```python
from build123d import *
from OCP.BRepAlgoAPI import BRepAlgoAPI_Cut
from OCP.TopTools import TopTools_ListOfShape

# Parameters (mm, degrees)
BOSS_EXTRUDE1_DEPTH   = 8
CUT_EXTRUDE2_DEPTH    = 3.1
CUT_EXTRUDE4_DEPTH    = 3.1
CUT_EXTRUDE6_START    = -3.1
CUT_EXTRUDE6_DEPTH    = 3.1
CUT_EXTRUDE7_START    = -3.1
CUT_EXTRUDE7_DEPTH    = 3.1
FILLET1_R             = 0.1
BODY_MOVE_COPY1_ANGLE = 89
BODY_MOVE_COPY3_ANGLE = 1
CUT_EXTRUDE8_DEPTH    = 19.406951047
CUT_EXTRUDE9_DEPTH    = 19.406951047
SKETCH20_W            = 16
SKETCH20_H            = 7.8
BOSS_EXTRUDE2_DEPTH   = 2.54
BOSS_EXTRUDE3_DEPTH   = 16


with BuildPart() as part:
    # Sketch1 → Boss-Extrude1 (new body)
    with BuildSketch(Plane.XY.offset(4)):
        with BuildLine():
            Line((-3.6, 0), (-3.6, -16))
            ThreePointArc((-3.6, -16), (0, -19.6), (3.6, -16))
            Line((3.6, -16), (3.6, 0))
            ThreePointArc((3.6, 0), (0, 3.6), (-3.6, 0))
        make_face()
    extrude(amount=-BOSS_EXTRUDE1_DEPTH)

    # Sketch3 → Cut-Extrude2 (cut)
    with BuildSketch(Plane.XY.offset(4)):
        with BuildLine():
            Line((2.8, -4.8), (2.8, -3.2))
            ThreePointArc((2.8, -3.2), (2.578885438, -2.842229124), (2.16, -2.88))
            ThreePointArc((2.16, -2.88), (0, -3.6), (-2.16, -2.88))
            ThreePointArc((-2.16, -2.88), (-2.578885438, -2.842229124), (-2.8, -3.2))
            Line((-2.8, -3.2), (-2.8, -4.8))
            ThreePointArc((-2.8, -4.8), (-2.578885438, -5.157770876), (-2.16, -5.12))
            ThreePointArc((-2.16, -5.12), (0, -4.4), (2.16, -5.12))
            ThreePointArc((2.16, -5.12), (2.578885438, -5.157770876), (2.8, -4.8))
        make_face()
    extrude(amount=-CUT_EXTRUDE2_DEPTH, mode=Mode.SUBTRACT)

    # Sketch5 → Cut-Extrude4 (cut)
    with BuildSketch(Plane.XY.offset(4)):
        with BuildLine():
            Line((2.8, -12.8), (2.8, -11.2))
            ThreePointArc((2.8, -11.2), (2.578885438, -10.842229124), (2.16, -10.88))
            ThreePointArc((2.16, -10.88), (0, -11.6), (-2.16, -10.88))
            ThreePointArc((-2.16, -10.88), (-2.578885438, -10.842229124), (-2.8, -11.2))
            Line((-2.8, -11.2), (-2.8, -12.8))
            ThreePointArc((-2.8, -12.8), (-2.578885438, -13.157770876), (-2.16, -13.12))
            ThreePointArc((-2.16, -13.12), (0, -12.4), (2.16, -13.12))
            ThreePointArc((2.16, -13.12), (2.578885438, -13.157770876), (2.8, -12.8))
        make_face()
    extrude(amount=-CUT_EXTRUDE4_DEPTH, mode=Mode.SUBTRACT)

    # Sketch7 → Cut-Extrude6 (cut)
    with BuildSketch(Plane(origin=(0, 0, -4), x_dir=(-1, 0, 0), z_dir=(0, 0, -1)).offset(CUT_EXTRUDE6_START)):
        with BuildLine():
            Line((2.8, -4.8), (2.8, -3.2))
            ThreePointArc((2.8, -3.2), (2.578885438, -2.842229124), (2.16, -2.88))
            ThreePointArc((2.16, -2.88), (0, -3.6), (-2.16, -2.88))
            ThreePointArc((-2.16, -2.88), (-2.578885438, -2.842229124), (-2.8, -3.2))
            Line((-2.8, -3.2), (-2.8, -4.8))
            ThreePointArc((-2.8, -4.8), (-2.578885438, -5.157770876), (-2.16, -5.12))
            ThreePointArc((-2.16, -5.12), (0, -4.4), (2.16, -5.12))
            ThreePointArc((2.16, -5.12), (2.578885438, -5.157770876), (2.8, -4.8))
        make_face()
    extrude(amount=CUT_EXTRUDE6_DEPTH, mode=Mode.SUBTRACT)

    # Sketch8 → Cut-Extrude7 (cut)
    with BuildSketch(Plane(origin=(0, 0, -4), x_dir=(-1, 0, 0), z_dir=(0, 0, -1)).offset(CUT_EXTRUDE7_START)):
        with BuildLine():
            Line((-2.8, -11.2), (-2.8, -12.8))
            ThreePointArc((-2.8, -12.8), (-2.578885438, -13.157770876), (-2.16, -13.12))
            ThreePointArc((-2.16, -13.12), (0, -12.4), (2.16, -13.12))
            ThreePointArc((2.16, -13.12), (2.578885438, -13.157770876), (2.8, -12.8))
            Line((2.8, -12.8), (2.8, -11.2))
            ThreePointArc((2.8, -11.2), (2.578885438, -10.842229124), (2.16, -10.88))
            ThreePointArc((2.16, -10.88), (0, -11.6), (-2.16, -10.88))
            ThreePointArc((-2.16, -10.88), (-2.578885438, -10.842229124), (-2.8, -11.2))
        make_face()
    extrude(amount=CUT_EXTRUDE7_DEPTH, mode=Mode.SUBTRACT)

    # Sketch10 → Cut-Revolve1 (revolve, cut)
    with BuildSketch(Plane(origin=(0, -16, 0), x_dir=(1, 0, 0), z_dir=(0, 1, 0))):
        Polygon((3.1, 4), (0, 4), (0, -4), (3.1, -4), (3.1, -3.2), (2.4, -3.2), (2.4, 3.2), (3.1, 3.2), align=None)
    revolve(axis=Axis((0, -16, -4), (0, 0, 1)), mode=Mode.SUBTRACT)

    # Sketch13 → Cut-Revolve4 (revolve, cut)
    with BuildSketch(Plane(origin=(0, 0, 0), x_dir=(1, 0, 0), z_dir=(0, 1, 0))):
        Polygon((3.1, 4), (0, 4), (0, -4), (3.1, -4), (3.1, -3.2), (2.4, -3.2), (2.4, 3.2), (3.1, 3.2), align=None)
    revolve(axis=Axis((0, 0, -4), (0, 0, 1)), mode=Mode.SUBTRACT)

    # Fillet1
    fillet1_edges = [part.edges().sort_by_distance(p)[0] for p in [
        (0, -19.6, -4),
        (3.6, -8, -4),
        (0, 3.6, -4),
        (3.6, -8, 4),
        (0, -19.6, 4),
        (-3.6, -8, 4),
        (0, 3.6, 4),
        (-3.6, -8, -4),
    ]]
    fillet(fillet1_edges, radius=FILLET1_R)


with BuildPart() as part_1:
    # Body-Move/Copy1: moved
    add(part.part.rotate(Axis((-1.61875778, -8, 0), (0, 0, 1)), BODY_MOVE_COPY1_ANGLE))


with BuildPart() as part_2:
    # Body-Move/Copy3: read off the stored shape, not the designer's step
    # Body-Move/Copy3: moved
    add(part_1.part.moved(Location((-0.0519755, -0.1124913, 0))).rotate(Axis((0, 0, 0), (0, 0, 1)), BODY_MOVE_COPY3_ANGLE))

    # Sketch14 → Cut-Extrude8 (cut, through all)
    with BuildSketch(Plane.XY.offset(4)):
        Polygon((-3.814896337, -5.759656314), (-3.814896337, -7.283656314), (-2.290892666, -7.283656314), (-2.290892666, -8.807656314), (-0.766892666, -8.807656314), (-0.766892666, -7.283656314), (0.757103663, -7.283656314), (0.757103663, -5.759656314), (-0.766892666, -5.759656314), (-0.766892666, -4.235656314), (-2.290892666, -4.235656314), (-2.290892666, -5.759656314), align=None)
    extrude(amount=-CUT_EXTRUDE8_DEPTH, mode=Mode.SUBTRACT)

    # Sketch15 → Cut-Extrude9 (cut, through all)
    with BuildSketch(Plane.XY.offset(4)):
        with BuildLine():
            Line((-2.290892666, -4.235656314), (-0.766892666, -4.235656314))
            Line((-0.766892666, -4.235656314), (-0.805995992, -4.222621872))
            ThreePointArc((-0.805995992, -4.222621872), (-1.528892666, -4.105311891), (-2.251789339, -4.222621872))
            Line((-2.251789339, -4.222621872), (-2.290892666, -4.235656314))
        make_face()
    extrude(amount=-CUT_EXTRUDE9_DEPTH, mode=Mode.SUBTRACT)


with BuildPart() as cirpattern1_tool:
    # CirPattern1: read off the stored shape, not the designer's step
    # CirPattern1: loft between two sections, ruled curve by curve
    cirpattern1_from = [
        Edge.make_three_point_arc((-3.827927108, -5.798759641, -4), (-3.945237088, -6.521656314, -4), (-3.827927108, -7.244552987, -4)),
        Edge.make_line((-3.827927108, -7.244552987, -4), (-3.814892666, -7.283656314, -4)),
        Edge.make_line((-3.827927108, -5.798759641, -4), (-3.814892666, -5.759656314, -4)),
        Edge.make_line((-3.814892666, -5.759656314, -4), (-3.814892666, -7.283656314, -4)),
    ]
    cirpattern1_to = [
        Edge.make_three_point_arc((-3.827927108, -5.798759641, 4), (-3.945237088, -6.521656314, 4), (-3.827927108, -7.244552987, 4)),
        Edge.make_line((-3.827927108, -7.244552987, 4), (-3.814892666, -7.283656314, 4)),
        Edge.make_line((-3.827927108, -5.798759641, 4), (-3.814892666, -5.759656314, 4)),
        Edge.make_line((-3.814892666, -5.759656314, 4), (-3.814892666, -7.283656314, 4)),
    ]
    cirpattern1 = Solid(Shell([*[Face.make_surface_from_curves(cirpattern1_from[k], cirpattern1_to[k]) for k in range(4)], Face(Wire(cirpattern1_from)), Face(Wire(cirpattern1_to))]))
    add(cirpattern1)


with BuildPart() as part_3:
    add(part_2.part)

    # CirPattern1: cut by cirpattern1_tool, with a tolerance
    cirpattern1_stock = TopTools_ListOfShape()
    cirpattern1_stock.Append(part_3.part.wrapped)
    cirpattern1_tools = TopTools_ListOfShape()
    cirpattern1_tools.Append(cirpattern1_tool.part.wrapped)
    cirpattern1_cut = BRepAlgoAPI_Cut()
    cirpattern1_cut.SetArguments(cirpattern1_stock)
    cirpattern1_cut.SetTools(cirpattern1_tools)
    cirpattern1_cut.SetFuzzyValue(0.00001)
    cirpattern1_cut.Build()
    add(Compound.cast(cirpattern1_cut.Shape()).solids(), mode=Mode.REPLACE)


with BuildPart() as cirpattern1_2_tool:
    # CirPattern1 2: loft between two sections, ruled curve by curve
    cirpattern1_2_from = [
        Edge.make_three_point_arc((-2.251789339, -8.820690756, -4), (-1.528892666, -8.938000737, -4), (-0.805995992, -8.820690756, -4)),
        Edge.make_line((-0.766892666, -8.807656314, -4), (-0.805995992, -8.820690756, -4)),
        Edge.make_line((-2.251789339, -8.820690756, -4), (-2.290892666, -8.807656314, -4)),
        Edge.make_line((-2.290892666, -8.807656314, -4), (-0.766892666, -8.807656314, -4)),
    ]
    cirpattern1_2_to = [
        Edge.make_three_point_arc((-2.251789339, -8.820690756, 4), (-1.528892666, -8.938000737, 4), (-0.805995992, -8.820690756, 4)),
        Edge.make_line((-0.766892666, -8.807656314, 4), (-0.805995992, -8.820690756, 4)),
        Edge.make_line((-2.251789339, -8.820690756, 4), (-2.290892666, -8.807656314, 4)),
        Edge.make_line((-2.290892666, -8.807656314, 4), (-0.766892666, -8.807656314, 4)),
    ]
    cirpattern1_2 = Solid(Shell([*[Face.make_surface_from_curves(cirpattern1_2_from[k], cirpattern1_2_to[k]) for k in range(4)], Face(Wire(cirpattern1_2_from)), Face(Wire(cirpattern1_2_to))]))
    add(cirpattern1_2)


with BuildPart() as part_4:
    add(part_3.part)

    # CirPattern1 2: cut by cirpattern1_2_tool, with a tolerance
    cirpattern1_2_stock = TopTools_ListOfShape()
    cirpattern1_2_stock.Append(part_4.part.wrapped)
    cirpattern1_2_tools = TopTools_ListOfShape()
    cirpattern1_2_tools.Append(cirpattern1_2_tool.part.wrapped)
    cirpattern1_2_cut = BRepAlgoAPI_Cut()
    cirpattern1_2_cut.SetArguments(cirpattern1_2_stock)
    cirpattern1_2_cut.SetTools(cirpattern1_2_tools)
    cirpattern1_2_cut.SetFuzzyValue(0.00001)
    cirpattern1_2_cut.Build()
    add(Compound.cast(cirpattern1_2_cut.Shape()).solids(), mode=Mode.REPLACE)


with BuildPart() as cirpattern1_3_tool:
    # CirPattern1 3: loft between two sections, ruled curve by curve
    cirpattern1_3_from = [
        Edge.make_three_point_arc((0.770141777, -7.244552987, -4), (0.887451757, -6.521656314, -4), (0.770141777, -5.798759641, -4)),
        Edge.make_line((0.757107334, -5.759656314, -4), (0.770141777, -5.798759641, -4)),
        Edge.make_line((0.770141777, -7.244552987, -4), (0.757103663, -7.283656314, -4)),
        Edge.make_line((0.757103663, -7.283656314, -4), (0.757107334, -5.759656314, -4)),
    ]
    cirpattern1_3_to = [
        Edge.make_three_point_arc((0.770141777, -7.244552987, 4), (0.887451757, -6.521656314, 4), (0.770141777, -5.798759641, 4)),
        Edge.make_line((0.757107334, -5.759656314, 4), (0.770141777, -5.798759641, 4)),
        Edge.make_line((0.770141777, -7.244552987, 4), (0.757107334, -7.283656314, 4)),
        Edge.make_line((0.757107334, -7.283656314, 4), (0.757107334, -5.759656314, 4)),
    ]
    cirpattern1_3 = Solid(Shell([*[Face.make_surface_from_curves(cirpattern1_3_from[k], cirpattern1_3_to[k]) for k in range(4)], Face(Wire(cirpattern1_3_from)), Face(Wire(cirpattern1_3_to))]))
    add(cirpattern1_3)


with BuildPart() as part_5:
    add(part_4.part)

    # CirPattern1 3: cut by cirpattern1_3_tool, with a tolerance
    cirpattern1_3_stock = TopTools_ListOfShape()
    cirpattern1_3_stock.Append(part_5.part.wrapped)
    cirpattern1_3_tools = TopTools_ListOfShape()
    cirpattern1_3_tools.Append(cirpattern1_3_tool.part.wrapped)
    cirpattern1_3_cut = BRepAlgoAPI_Cut()
    cirpattern1_3_cut.SetArguments(cirpattern1_3_stock)
    cirpattern1_3_cut.SetTools(cirpattern1_3_tools)
    cirpattern1_3_cut.SetFuzzyValue(0.00001)
    cirpattern1_3_cut.Build()
    add(Compound.cast(cirpattern1_3_cut.Shape()).solids(), mode=Mode.REPLACE)

    # Sketch20 → Boss-Extrude2 (add)
    with BuildSketch(Plane.XZ.offset(10.121656314)):
        with Locations((-1.528896337, 0)):
            Rectangle(SKETCH20_W, SKETCH20_H)
    extrude(amount=BOSS_EXTRUDE2_DEPTH)

    # Sketch23 → Boss-Extrude3 (add)
    with BuildSketch(Plane(origin=(6.471103663, 0, 0), x_dir=(0, 0, -1), z_dir=(1, 0, 0))):
        Polygon((-3.9, -12.661656314), (50.879562339, -67.441218652), (58.679562339, -64.901218652), (3.9, -10.121656314), align=None)
    extrude(amount=-BOSS_EXTRUDE3_DEPTH)


solid = part_5.part
```
The model under review builds one solid part; all positions refer to its coordinate system, in mm. A direction names the side the tool comes from. Round coordinates to 2 decimals unless told otherwise and drop trailing zeros. Write each loop counter-clockwise with the first axis right and the second up, starting at its lowest first coordinate (ties: lowest second). Pieces come first, ordered by that corner, then holes. Notation, with made-up numbers: (53.5, -14.75) -> (95.5, -14.75) arc R14 cw to (95.5, 4.25) -> close; hole circle Ø2 at (-32, 24.25). An arc over 180 degrees is marked (long way). Use CSV: the item, a comma, the result in double quotes.
Q1. To check wall thickness, follow probe 1 along X at (y, z) = (-33, -25); probe 2 along Y at (x, z) = (-1, -2.5); probe 3 along Y at (x, z) = (-10.5, 0). State the ranges of each line that lie inside material, in increasing order. Write a range as [from, to].
Checks:
probe 1,"[-9.53, 6.47]"
probe 2,"[-19.06, -8.88], [-4.17, -2.92]"
probe 3,"[-9.99, -8.72], [-4.33, -3.06]"
Q2. Consider section A-A (y = -34.5). Give the boundary of the cut face in (x, z).
Checks:
outline,"(-9.53, -28.28) -> (6.47, -28.28) -> (6.47, -17.94) -> (-9.53, -17.94) -> close"
Q3. For faces 1 (the flat face through (-2.291, -8, 0)), 2 (the flat face through (-6, -9.322, -2)), 3 (the cylindrical face through (9.22, -5.09, 3.59)), list the 3-axis set-ups (+Z, -Z, +X, -X, +Y, -Y) from which the entire face can be reached by the end or side of a thin tool; tool diameter is ignored.
Checks:
face 1,"+Z, -Z"
face 2,"-Z"
face 3,"+Z"
Q4. For pin 1 Ø10 at (x, z) = (-6.5, -23) entering from -Y; pin 2 Ø3 at (x, y) = (-8, -25.5) entering from -Z; pin 3 Ø1.7 at (y, z) = (-8, 1.5) entering from +X, all flat-tipped, find the tip position at first contact; note any pin that passes through.
Checks:
pin 1,"y = -44.56"
pin 2,"z = -20.78"
pin 3,"x = 10.02"
Q5. Consider section B-B (z = -30). Give the boundary of the cut face in (x, y).
Checks:
outline,"(-9.53, -46.56) -> (6.47, -46.56) -> (6.47, -36.22) -> (-9.53, -36.22) -> close"
